Part print with two shaded views. Sizes in mm from the minimum x, y, z corner. Round coordinates to 2 decimals unless told otherwise and drop trailing zeros. Loops run counter-clockwise (first coordinate to the right, second up) from the corner with the lowest first, then second, coordinate; pieces in that order, holes last. Notation, with made-up numbers: (17.25, -30.75) -> (61.25, -30.75) arc R26 cw to (61.25, 8.25) -> close; hole circle Ø3 at (-20.75, 21). An arc over 180 degrees is marked (long way). Answer as a JSON object with one key per item and string values. Group by question number.
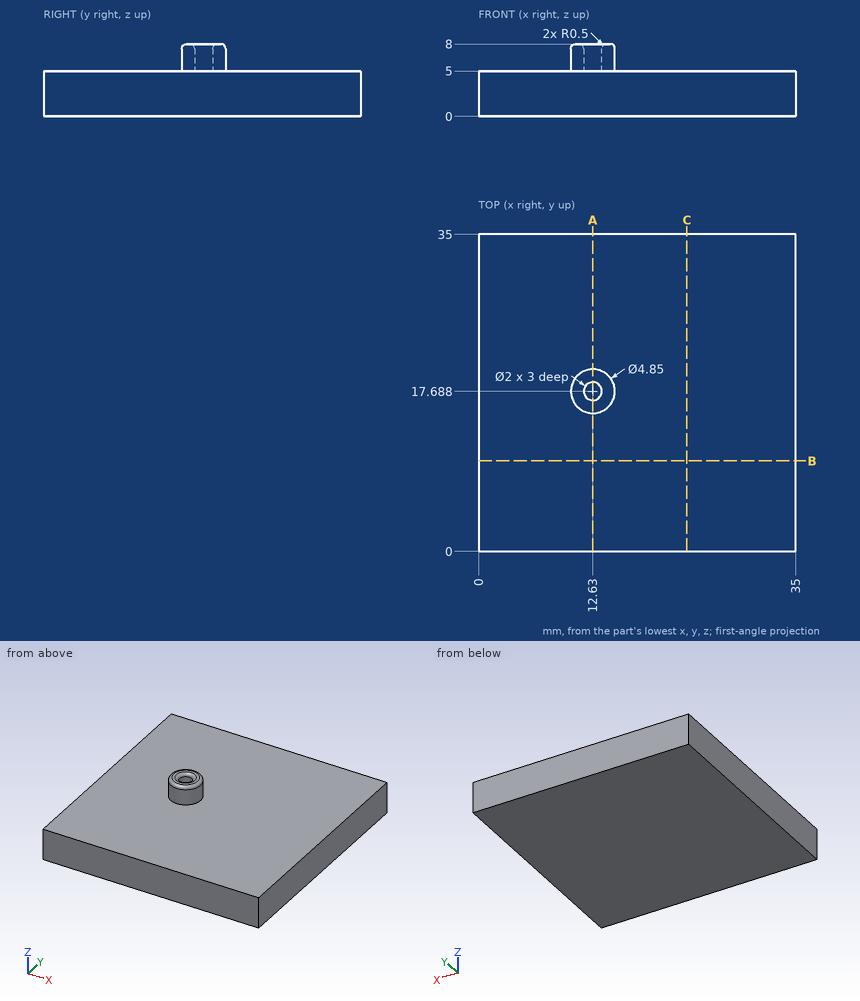
Item 1: Band-saw the part on B-B, the plane y = 10. List the corners of the cut face in (x, z), plus the area to 3 significant figures.
Item 2: Drop flat-ended pins along their axis: pin 1 Ø2 at (x, z) = (11.5, 5) entering from -Y; pin 2 Ø0.6 at (x, y) = (12.5, 17.5) entering from +Z. Give the stop position or say it passes through.
Item 3: Drill centre lines: line 1 (Y direction, x = 12.63, z = 6.15); line 2 (Z direction, x = 31, y = 16.5); line 3 (X direction, y = 17, z = 6.75) (1 decimal). Where is each one in solid material? Low to high.
Item 4: Band-saw the part on A-A, the plane x = 12.63. List the corners of the cut face in (y, z).
Entries:
{
 "1": {"outline": "(0, 0) -> (35, 0) -> (35, 5) -> (0, 5) -> close", "area": "175 mm²"},
 "2": {"pin 1": "y = 0", "pin 2": "z = 5"},
 "3": {"line 1": "15.26 to 16.69, 18.69 to 20.11", "line 2": "0 to 5", "line 3": "10.3 to 11.9, 13.4 to 15"},
 "4": {"outline": "(0, 0) -> (35, 0) -> (35, 5) -> (20.11, 5) -> (20.11, 7.5) arc R0.5 ccw to (19.61, 8) -> (19.19, 8) arc R0.5 ccw to (18.69, 7.5) -> (18.69, 5) -> (16.69, 5) -> (16.69, 7.5) arc R0.5 ccw to (16.19, 8) -> (15.76, 8) arc R0.5 ccw to (15.26, 7.5) -> (15.26, 5) -> (0, 5) -> close"}
}
